Design review of the part built by this model. Coordinates are the model's own, in mm. Face numbers are marked on the shaded views. Give positions to 0.01 mm unless a question says otherwise; leave off trailing zeros. Loops run counter-clockwise (first coordinate to the right, second up) from the corner with the lowest first, then second, coordinate; pieces in that order, holes last.
from build123d import *

# Parameters (mm, degrees)
F0_W     = 75
F0_H     = 25
F0_R     = 5
F1_DEPTH = 3
F0_W_2   = 85
F0_H_2   = 35
F2_DEPTH = 3
F3_W     = 85
F3_H     = 35
F3_W_2   = 81
F3_H_2   = 31
F4_DEPTH = 5


with BuildPart() as f1:
    # F0 (on Top) → F1 (new body)
    with BuildSketch(Plane.XY):
        with Locations((0.065177, 0.136048)):
            Rectangle(F0_W, F0_H)
        with Locations((-24.984823, 0.182369)):
            Circle(F0_R, mode=Mode.SUBTRACT)
        with Locations((-8.284823, 0.182369)):
            Circle(F0_R, mode=Mode.SUBTRACT)
        with Locations((8.415177, 0.182369)):
            Circle(F0_R, mode=Mode.SUBTRACT)
        with Locations((25.115177, 0.182369)):
            Circle(F0_R, mode=Mode.SUBTRACT)
    extrude(amount=F1_DEPTH)

    # F0 (on Top) → F2 (join)
    with BuildSketch(Plane.XY):
        with Locations((0.065177, 0.136048)):
            Rectangle(F0_W_2, F0_H_2)
        with Locations((0.065177, 0.136048)):
            Rectangle(F0_W, F0_H, mode=Mode.SUBTRACT)
    extrude(amount=F2_DEPTH)

    # F3 (on face) → F4 (join)
    with BuildSketch(Plane(origin=(0, 0, 0), x_dir=(1, 0, 0), z_dir=(0, 0, -1))):
        with Locations((0.065177, -0.136048)):
            Rectangle(F3_W, F3_H)
        with Locations((0.065177, -0.136048)):
            Rectangle(F3_W_2, F3_H_2, mode=Mode.SUBTRACT)
    extrude(amount=F4_DEPTH)


solid = f1.part
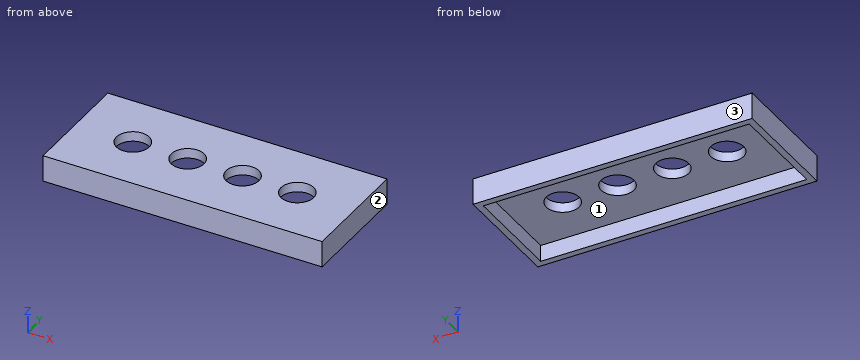
Q1. Take a section at A-A (z = -1.75). Give the boundary of the cut face in (x, y), plus the area to 3 significant figures.
Results:
outline: (-42.43, -17.36) - (42.57, -17.36) - (42.57, 17.64) - (-42.43, 17.64) - close; hole (-40.43, -15.36) - (40.57, -15.36) - (40.57, 15.64) - (-40.43, 15.64) - close
area: 464 mm2
Q2. Wall thickness on line 1 (X direction, y = -4, z = -3.5); line 2 (Y direction, x = 19, z = -3.5); line 3 (X direction, y = -2, z = 2): over which ranges is each line inside the solid? List them lowest first.
Results:
line 1: x = -42.43 to -40.43, 40.57 to 42.57
line 2: y = -17.36 to -15.36, 15.64 to 17.64
line 3: x = -42.43 to -29.48, -20.49 to -12.78, -3.79 to 3.92, 12.91 to 20.62, 29.61 to 42.57
Q3. Take a section at C-C (y = 6). Give the boundary of the cut face in (x, z), plus the area to 3 significant figures.
Results:
outline: (-42.43, -5) - (-40.43, -5) - (-40.43, 0) - (40.57, 0) - (40.57, -5) - (42.57, -5) - (42.57, 3) - (-42.43, 3) - close
area: 275 mm2
Q4. Take a section at B-B (x = 10). Give the boundary of the cut face in (y, z), plus the area to 3 significant figures.
Results:
outline: (-17.36, -5) - (-15.36, -5) - (-15.36, 0) - (-4.56, 0) - (-4.56, 3) - (-17.36, 3) - close; (4.92, 0) - (15.64, 0) - (15.64, -5) - (17.64, -5) - (17.64, 3) - (4.92, 3) - close
area: 96.5 mm2
Q5. Take a section at D-D (x = 0.5). Give the boundary of the cut face in (y, z).
Results:
outline: (-17.36, -5) - (-15.36, -5) - (-15.36, 0) - (15.64, 0) - (15.64, -5) - (17.64, -5) - (17.64, 3) - (-17.36, 3) - close
Q6. Insertion check: pin 1 (8 mm diameter, centred on x = -10.5, y = 1.5, fed in from -Z); pin 2 (8 mm diameter, centred on x = -24.98, y = 0.18, fed in from -Z). Each pin has a flat end and moves straight along its axis. Give the tip position at first contact, or say it passes through.
Results:
pin 1: stops at z = 0
pin 2: passes through
Q7. Draft analysis for pull direction Y (two halves, no side actions). For the marked faces 1, 2 and 3, state which applies: pulls with the +Y half, pulls with the -Y half, needs draft (parallel to the pull), parting line crosses it, or undercut.
Results:
face 1: undercut
face 2: needs draft
face 3: pulls with the +Y half
